```python
from build123d import *

# Parameters (mm, degrees)
BOSS_EXTRUDE1_DEPTH = 2.54


with BuildPart() as part:
    # Sketch1 → Boss-Extrude1 (new body)
    with BuildSketch(Plane.XY):
        with BuildLine():
            Line((-58.91868881, 27.487867139), (-76.2, -76.2))
            ThreePointArc((-76.2, -76.2), (-68.819471722, -87.89820202), (-56.352718657, -81.906524778))
            Line((-56.352718657, -81.906524778), (-53.975, -76.2))
            Line((-53.975, -76.2), (-41.356410256, -45.915384615))
            ThreePointArc((-41.356410256, -45.915384615), (-36.678025825, -40.232961262), (-29.633333333, -38.1))
            Line((-29.633333333, -38.1), (29.633333333, -38.1))
            ThreePointArc((29.633333333, -38.1), (36.678025825, -40.232961262), (41.356410256, -45.915384615))
            Line((41.356410256, -45.915384615), (53.975, -76.2))
            Line((53.975, -76.2), (56.352718657, -81.906524778))
            ThreePointArc((56.352718657, -81.906524778), (68.819471722, -87.89820202), (76.2, -76.2))
            Line((76.2, -76.2), (58.91868881, 27.487867139))
            ThreePointArc((58.91868881, 27.487867139), (54.600447158, 35.090353777), (46.391485978, 38.1))
            Line((46.391485978, 38.1), (-46.391485978, 38.1))
            ThreePointArc((-46.391485978, 38.1), (-54.600447158, 35.090353777), (-58.91868881, 27.487867139))
        make_face()
    extrude(amount=BOSS_EXTRUDE1_DEPTH)


solid = part.part
```
Read the model definition and answer for the solid it produces. Units are mm, in the model's axes. A direction names the side the tool comes from. Coordinates: 2 decimals unless noted, no trailing zeros. Order: outer loops, then holes, each group sorted by start corner. A loop starts at its lowest first (then second) coordinate and runs counter-clockwise, first axis right, second up. Notation, with made-up numbers: (59, 16.5) - (95, 16.5) arc R36 ccw to (95, 51.5) - close; hole circle Ø10 at (67.25, 52.25). An arc over 180 degrees is marked (long way). Answer as a JSON object with one key per item and string values. Group by question number.
Item 1: Consider probe 1 along X at (y, z) = (-73, 0.45); probe 2 along X at (y, z) = (-51, 1.05) (3 decimals); probe 3 along Y at (x, z) = (-15.5, 0.65). Determine where each line is inside the solid, lowest interval first. Write a range as from..to.
Item 2: Section B-B (z = 1.2) is taken. Give the vertices of the cut face in (x, y) (3 decimals).
Item 3: The mould has two halves that part along X. Classify faces 3 (the face through (54.695, 35.009, 1.252)), 4 (the face through (-67.44, -23.63, 1.25)), 5 (the face through (68.615, -87.955, 1.252)): +X half, -X half, draft (parallel to the pull), parting line (faces both ways), or undercut.
Item 4: Section D-D (x = -49.5) is taken. Give the vertices of the cut face in (y, z), plus the area to 3 significant figures.
Item 5: Section C-C (y = 4.5) is taken. Give the vertices of the cut face in (x, z), plus the area to 3 significant figures.
Item 6: Flat-ended cylindrical pins translate along their axes: P1, Ø1, axis at x = 52.5, z = 2, coming from the +Y side; P2, Ø1, axis at y = -48, z = 1, coming from the +X side; P3, Ø1, axis at x = -54, y = -9, coming from the -Z side. Find the tip coordinate at first contact, or state that the pin passes through.
Item 7: Section A-A (y = -61.5) is taken. Give the vertices of the cut face in (x, z).
Item 8: A tool of negligible diameter and unlimited length cuts with its end or side. For faces 1 (the face through (-36.76, -40.29, 1.25)), 2 (the face through (67.68, -25.08, 1.25)), from which of +Z, -Z, +X, -X, +Y, -Y can it reach the whole face along a straight path? Write none if from no direction.
Results are:
{
 "1": {"probe 1": "x = -75.67..-52.64, 52.64..75.67", "probe 2": "x = -72..-43.475, 43.475..72", "probe 3": "y = -38.1..38.1"},
 "2": {"outline": "(-76.2, -76.2) arc R10.394 ccw to (-56.353, -81.907) - (-41.356, -45.915) arc R12.7 cw to (-29.633, -38.1) - (29.633, -38.1) arc R12.7 cw to (41.356, -45.915) - (56.353, -81.907) arc R10.394 ccw to (76.2, -76.2) - (58.919, 27.488) arc R12.7 ccw to (46.391, 38.1) - (-46.391, 38.1) arc R12.7 ccw to (-58.919, 27.488) - close"},
 "3": {"face 3": "+X half", "face 4": "-X half", "face 5": "undercut"},
 "4": {"outline": "(-65.46, 0) - (37.71, 0) - (37.71, 2.54) - (-65.46, 2.54) - close", "area": "262 mm^2"},
 "5": {"outline": "(-62.75, 0) - (62.75, 0) - (62.75, 2.54) - (-62.75, 2.54) - close", "area": "319 mm^2"},
 "6": {"P1": "stops at y = 36.79", "P2": "stops at x = 71.58", "P3": "stops at z = 0"},
 "7": {"outline": "(-73.75, 0) - (-47.85, 0) - (-47.85, 2.54) - (-73.75, 2.54) - close; (47.85, 0) - (73.75, 0) - (73.75, 2.54) - (47.85, 2.54) - close"},
 "8": {"face 1": "+Z, -Z, -Y", "face 2": "+Z, -Z, +X, +Y"}
}
